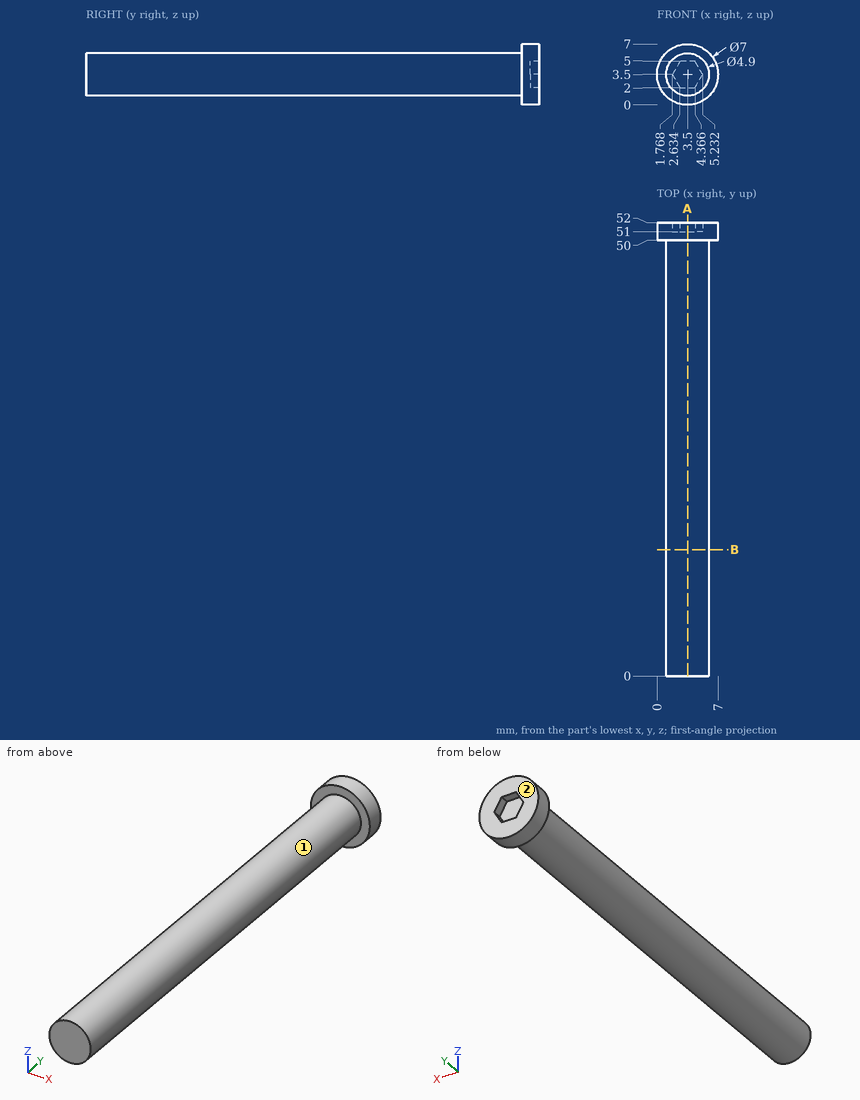
Input: dimensioned drawing with shaded views. Units: mm. Origin: part minimum x, y, z. A direction names the side the tool comes from. Coordinates: 2 decimals unless noted, no trailing zeros. Loops run counter-clockwise (first coordinate to the right, second up) from the corner with the lowest first, then second, coordinate; pieces in that order, holes last. Notation, with made-up numbers: M 50,10 L 93,10 A11 ccw 93,19 Z; hole C 0,48 d1. An arc over 180 degrees is marked long. Put each result on its own line as item: value.
(1) Access query for the marked faces 1 and 2. Directions: +Z, -Z, +X, -X, +Y, -Y. A direction counts if a zero-diameter tool reaches every point of the face in a straight line with its end or side. Return the directions, or none.
Answer sheet:
face 1: -Y
face 2: +Z, -Z, +X, -X, +Y
(2) Cut plane B-B on y = 14.5. Return the cut outline in (x, z), then the cut area to 3 significant figures.
Answer sheet:
outline: C 3.5,3.5 d4.9
area: 18.9 mm^2
(3) First-contact query: pin 1 (2 mm diameter, centred on x = 3.5, y = 45, fed in from -Z); pin 2 (0.5 mm diameter, centred on x = 3, y = 51.5, fed in from +Z); pin 3 (4 mm diameter, centred on x = 3.5, y = 28.5, fed in from +Z). Flat tips, straight axial feed; report the tip coordinate or a pass-through.
Answer sheet:
pin 1: stops at z = 1.05
pin 2: stops at z = 6.99
pin 3: stops at z = 5.95
(4) Cut plane A-A on x = 3.5. Return the cut outline in (y, z).
Answer sheet:
outline: M 0,1.05 L 50,1.05 L 50,0 L 52,0 L 52,2 L 51,2 L 51,5 L 52,5 L 52,7 L 50,7 L 50,5.95 L 0,5.95 Z
(5) Material intervals for probe 1 along Y at (x, z) = (5.75, 1.5); probe 2 along Y at (x, z) = (4, 3.5); probe 3 along Z at (x, y) = (4, 45), sorted ascending.
Answer sheet:
probe 1: y = 50 to 52
probe 2: y = 0 to 51
probe 3: z = 1.1 to 5.9
